Geometry check sheet. Reference: drawing and pictorial views, mm from the part's lowest x, y, z. A direction names the side the tool comes from. Coordinates: 2 decimals unless noted, no trailing zeros. Loops run counter-clockwise (first coordinate to the right, second up) from the corner with the lowest first, then second, coordinate; pieces in that order, holes last. Notation, with made-up numbers: M 32.25,-37 L 48.25,-37 A10 cw 48.25,-18 Z; hole C 44.5,60 d6. An arc over 180 degrees is marked long. Write item = value, one per line. Start each with the question number.
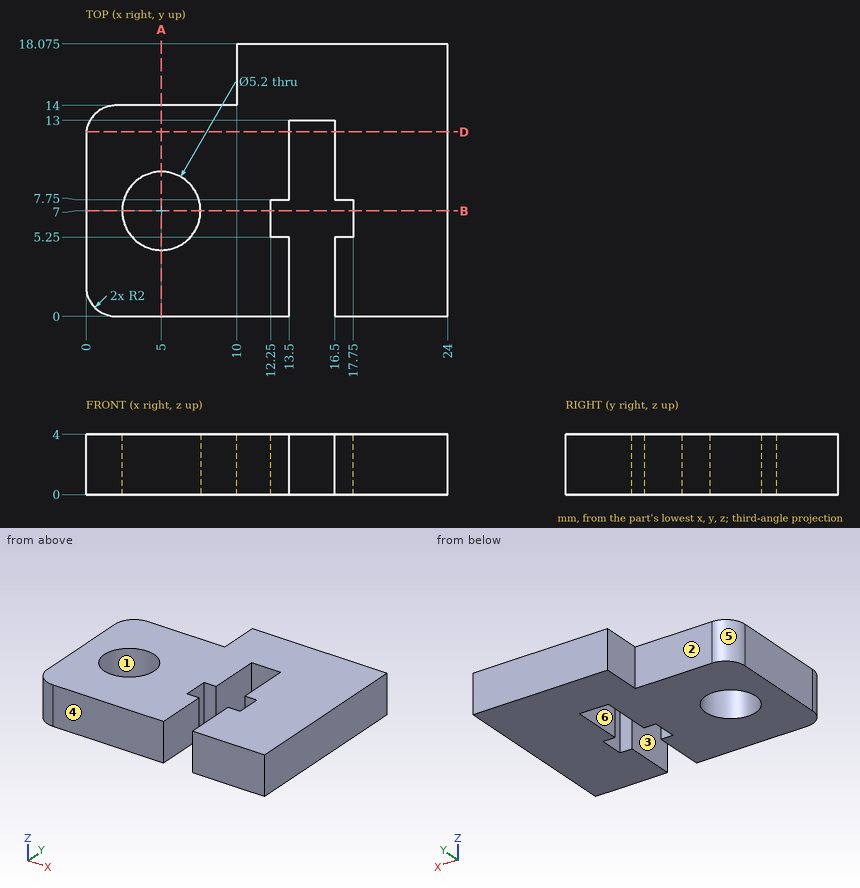
Q1. Gauge pin test, flat ends, axial feed: pin 1 (8 mm diameter, centred on x = 5, y = 11, fed in from -Z); pin 2 (0.9 mm diameter, centred on x = 15, z = 2.5, fed in from -Y); pin 3 (2 mm diameter, centred on x = 3, z = 1.5, fed in from +Y); pin 4 (1.2 mm diameter, centred on y = 15.5, z = 2, fed in from -X). Record the tip position at first contact, or that the pin passes through.
Q2. Scan lines: L1, parallel to Y at x = 5, z = 3.2; L2, parallel to X at y = 9.75, z = 2.9; L3, parallel to X at y = 6.75, z = 1. Record each from-to range of solid material in increasing order. Write a range as [from, to].
Q3. Sectioned sample at D-D on y = 12.25. Record the cut outline in (x, z).
Q4. Set-up check for the marked faces 1, 2 and 3: record each of +Z, -Z, +X, -X, +Y, -Y from which the full face is reachable in a straight line by a thin tool's end or side.
Q5. Sectioned sample at A-A on x = 5. Record the cut outline in (y, z), plus the area to 3 significant figures.
Q6. Sectioned sample at B-B on y = 7. Record the cut outline in (x, z), plus the area to 3 significant figures.
Q7. Mould release check, pull along X, two halves, no side actions. Record for the marked faces 4, 5 and 6: +X half, -X half, draft (parallel to the pull), parting line (faces both ways), or undercut.
Solutions:
q1.pin_1 = 0
q1.pin_2 = 13
q1.pin_3 = 14
q1.pin_4 = 10
q2.L1 = [0, 4.4], [9.6, 14]
q2.L2 = [0, 13.5], [16.5, 24]
q2.L3 = [0, 2.41], [7.59, 12.25], [17.75, 24]
q3.outline = M 0.02,0 L 13.5,0 L 13.5,4 L 0.02,4 Z; M 16.5,0 L 24,0 L 24,4 L 16.5,4 Z
q4.face_1 = +Z, -Z
q4.face_2 = +Z, -Z, -X, +Y
q4.face_3 = +Z, -Z, -Y
q5.outline = M 0,0 L 4.4,0 L 4.4,4 L 0,4 Z; M 9.6,0 L 14,0 L 14,4 L 9.6,4 Z
q5.area = 35.2 mm²
q6.outline = M 0,0 L 2.4,0 L 2.4,4 L 0,4 Z; M 7.6,0 L 12.25,0 L 12.25,4 L 7.6,4 Z; M 17.75,0 L 24,0 L 24,4 L 17.75,4 Z
q6.area = 53.2 mm²
q7.face_4 = draft
q7.face_5 = -X half
q7.face_6 = undercut
